Print and shaded views of the part. All mm, measured from the part's lowest x, y and z. A direction names the side the tool comes from. Give positions to 0.01 mm unless a question says otherwise; leave off trailing zeros. Order: outer loops, then holes, each group sorted by start corner. A loop starts at its lowest first (then second) coordinate and runs counter-clockwise, first axis right, second up. Notation, with made-up numbers: (54.25, 81.25) - (105.25, 81.25) arc R16 ccw to (105.25, 104.25) - close; hole circle Ø10 at (69, -4). An arc over 180 degrees is marked (long way). Answer in a Markdown table with one row per item.
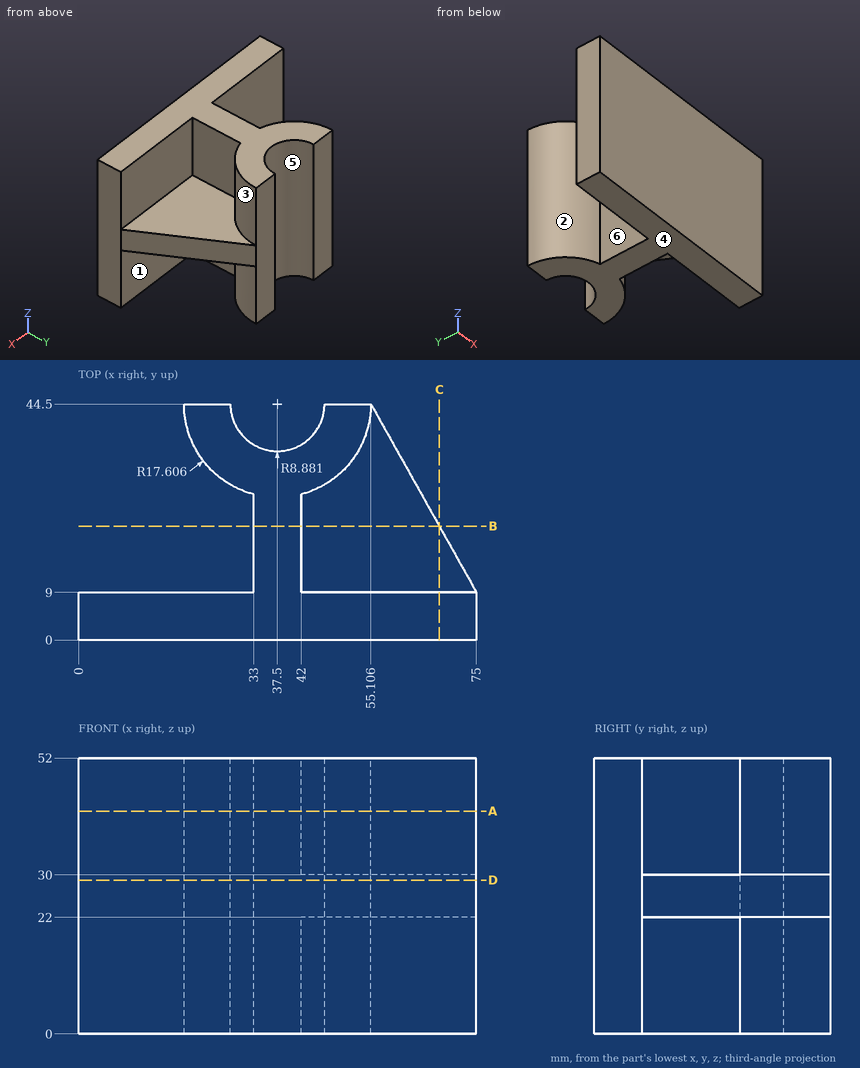
1. Cut at D-D on z = 29. Write the cut outline in (x, y), and give its area (3 significant figures).
Check result:
| item | result |
|---|---|
| outline | (0, 0) - (75, 0) - (75, 9) - (55.11, 44.5) - (46.38, 44.5) arc R8.88 cw to (28.62, 44.5) - (19.89, 44.5) arc R17.61 ccw to (33, 27.48) - (33, 9) - (0, 9) - close |
| area | 1,850 mm² |
2. Two-plate mould, pull along Y, no slides. Class the marked faces 4, 5 and 6: +Y half, -Y half, draft (parallel to the pull), parting line (faces both ways), or undercut.
Check result:
| item | result |
|---|---|
| face 4 | draft |
| face 5 | +Y half |
| face 6 | undercut |
3. Cut at B-B on y = 21.5. Write the cut outline in (x, z) (3 decimals).
Check result:
| item | result |
|---|---|
| outline | (33, 0) - (42, 0) - (42, 22) - (67.995, 22) - (67.995, 30) - (42, 30) - (42, 52) - (33, 52) - close |
4. Cut at C-C on x = 68. Write the cut outline in (y, z), and give its area (3 significant figures).
Check result:
| item | result |
|---|---|
| outline | (0, 0) - (9, 0) - (9, 22) - (21.49, 22) - (21.49, 30) - (9, 30) - (9, 52) - (0, 52) - close |
| area | 568 mm² |
5. Which spindle directions (+Z, -Z, +X, -X, +Y, -Y) get a long thin tool onto all of the face, cutting with end or side? Do the marked faces 1, 2 and 3. Say none if no direction does.
Check result:
| item | result |
|---|---|
| face 1 | -Z, +X |
| face 2 | +Z, -Z, -X |
| face 3 | +Z, +X |
6. Cut at A-A on z = 42. Write the cut outline in (x, y), and give its area (3 significant figures).
Check result:
| item | result |
|---|---|
| outline | (0, 0) - (75, 0) - (75, 9) - (42, 9) - (42, 27.48) arc R17.61 ccw to (55.11, 44.5) - (46.38, 44.5) arc R8.88 cw to (28.62, 44.5) - (19.89, 44.5) arc R17.61 ccw to (33, 27.48) - (33, 9) - (0, 9) - close |
| area | 1,200 mm² |
7. Probe line 1 (X direction, y = 12, z = 13); line 2 (Y direction, x = 19.5, z = 10.5); line 3 (Y direction, x = 25, z = 48). List the from-to ranges inside material, lowest first.
Check result:
| item | result |
|---|---|
| line 1 | x = 33 to 42 |
| line 2 | y = 0 to 9 |
| line 3 | y = 0 to 9, 32.1 to 44.5 |
8. Drop flat-ended pins along their axis: P1, Ø4, axis at y = 29, z = 23, coming from the +X side; P2, Ø9, axis at y = 15.5, z = 37.5, coming from the +X side; P3, Ø5.5, axis at y = 21.5, z = 18, coming from the -X side. Give the stop position or say it passes through.
Check result:
| item | result |
|---|---|
| P1 | stops at x = 64.91 |
| P2 | stops at x = 42 |
| P3 | stops at x = 33 |
